Can you work these out from the drawing? Everything is in mm from the part's minimum corner. Round coordinates to 2 decimals unless told otherwise and drop trailing zeros. Loops run counter-clockwise (first coordinate to the right, second up) from the corner with the lowest first, then second, coordinate; pieces in that order, holes last. Notation, with made-up numbers: (-4, 64.25) -> (35, 64.25) arc R25 ccw to (35, 81.25) -> close; hole circle Ø6 at (-13.75, -10). An arc over 180 degrees is marked (long way). Answer as a JSON object with one key per item and string values.
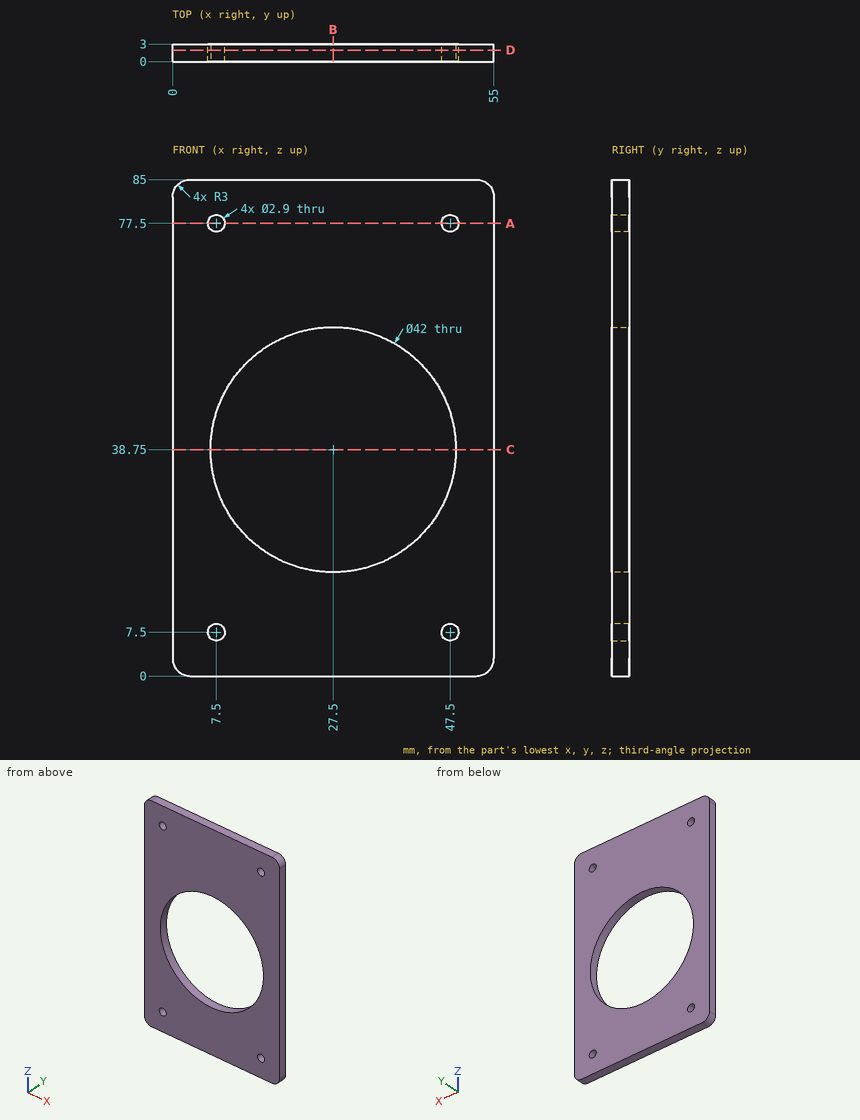
Q1. If I drill on L1, parallel to X at y = 1.9, z = 77.5; L2, parallel to X at y = 1.45, z = 38.75; L3, parallel to Z at x = 21, y = 2.75, over which ranges is the centre line in solid material (lowest first)? Write a range as [from, to].
Determined:
{"L1": "[0, 6.05], [8.95, 46.05], [48.95, 55]", "L2": "[0, 6.5], [48.5, 55]", "L3": "[0, 18.78], [58.72, 85]"}
Q2. I want a section at C-C, the plane z = 38.75. Write out the boundary of the cut face in (x, y), then the cut area to 3 significant figures.
Determined:
{"outline": "(0, 0) -> (6.5, 0) -> (6.5, 3) -> (0, 3) -> close; (48.5, 0) -> (55, 0) -> (55, 3) -> (48.5, 3) -> close", "area": "39.0 mm²"}
Q3. I'm going to push a flat-ended pin straight in: pin 1 (1.7 mm diameter, centred on x = 7.5, z = 7.5, fed in from +Y). Where does the tip first touch, or does it pass through?
Determined:
{"pin 1": "through"}
Q4. I want a section at B-B, the plane x = 27.5. Write out the boundary of the cut face in (y, z).
Determined:
{"outline": "(0, 0) -> (3, 0) -> (3, 17.75) -> (0, 17.75) -> close; (0, 59.75) -> (3, 59.75) -> (3, 85) -> (0, 85) -> close"}
Q5. I want a section at D-D, the plane y = 1.95. Write out the boundary of the cut face in (x, z), then the cut area to 3 significant figures.
Determined:
{"outline": "(0, 3) arc R3 ccw to (3, 0) -> (52, 0) arc R3 ccw to (55, 3) -> (55, 82) arc R3 ccw to (52, 85) -> (3, 85) arc R3 ccw to (0, 82) -> close; hole circle Ø2.9 at (7.5, 7.5); hole circle Ø2.9 at (7.5, 77.5); hole circle Ø42 at (27.5, 38.75); hole circle Ø2.9 at (47.5, 7.5); hole circle Ø2.9 at (47.5, 77.5)", "area": "3,260 mm²"}
Q6. I want a section at A-A, the plane z = 77.5. Write out the boundary of the cut face in (x, y).
Determined:
{"outline": "(0, 0) -> (6.05, 0) -> (6.05, 3) -> (0, 3) -> close; (8.95, 0) -> (46.05, 0) -> (46.05, 3) -> (8.95, 3) -> close; (48.95, 0) -> (55, 0) -> (55, 3) -> (48.95, 3) -> close"}
